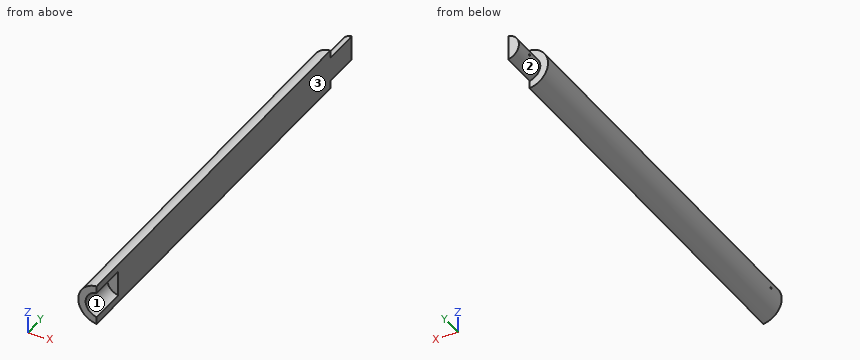
```python
from build123d import *

# Parameters (mm, degrees)
BOSS_EXTRUDE1_DEPTH     = 216.66667
BOSS_EXTRUDE2_START     = 216.66667
BOSS_EXTRUDE2_DEPTH     = 19.8
CUT_EXTRUDE2_START      = -1.4
SKETCH4_R               = 0.5
CUT_EXTRUDE2_DEPTH      = 9
SKETCH6_R               = 7
CUT_EXTRUDE3_DEPTH      = 20
CUT_EXTRUDE4_DEPTH      = 237.977817671
CUT_EXTRUDE4_DEPTH_BACK = 20
SKETCH7_R               = 0.5
CUT_EXTRUDE5_DEPTH      = 237.97781768
CUT_EXTRUDE5_DEPTH_BACK = 237.97781768
SKETCH10_R              = 0.5
CUT_EXTRUDE6_DEPTH      = 237.97781768
CUT_EXTRUDE6_DEPTH_BACK = 237.97781768
SKETCH11_W              = 3.5
SKETCH11_H              = 216.66667
CUT_EXTRUDE7_DEPTH      = 237.975709212
CUT_EXTRUDE7_DEPTH_BACK = 237.975709212
SKETCH12_W              = 3.499316008
SKETCH12_H              = 20


with BuildPart() as part:
    # Sketch1 → Boss-Extrude1 (new body)
    with BuildSketch(Plane(origin=(0, 0, 0), x_dir=(1, 0, 0), z_dir=(0, 1, 0))):
        with BuildLine():
            Line((0, 11), (0, -11))
            ThreePointArc((0, -11), (-11, 0), (0, 11))
        make_face()
    extrude(amount=BOSS_EXTRUDE1_DEPTH)

    # Sketch2 → Boss-Extrude2 (add)
    with BuildSketch(Plane(origin=(0, 0, 0), x_dir=(1, 0, 0), z_dir=(0, 1, 0)).offset(BOSS_EXTRUDE2_START)):
        with BuildLine():
            Line((0, 6.8), (0, -6.8))
            ThreePointArc((0, -6.8), (-6.8, 0), (0, 6.8))
        make_face()
    extrude(amount=BOSS_EXTRUDE2_DEPTH)

    # Sketch4 → Cut-Extrude2 (cut)
    with BuildSketch(Plane(origin=(0, 0, 0), x_dir=(0, 0, -1), z_dir=(1, 0, 0)).offset(CUT_EXTRUDE2_START)):
        with Locations((0, 226.66667)):
            Circle(SKETCH4_R)
    extrude(amount=-CUT_EXTRUDE2_DEPTH, mode=Mode.SUBTRACT)

    # Sketch6 → Cut-Extrude3 (cut)
    with BuildSketch(Plane(origin=(0, 0, 0), x_dir=(1, 0, 0), z_dir=(0, 1, 0))):
        Circle(SKETCH6_R)
    extrude(amount=CUT_EXTRUDE3_DEPTH, mode=Mode.SUBTRACT)

    # Sketch7 → Cut-Extrude4 (cut, two sides: drawn at the far end of the back side and taken through both)
    with BuildSketch(Plane(origin=(0, 0, 0), x_dir=(0, 0, -1), z_dir=(1, 0, 0)).offset(-CUT_EXTRUDE4_DEPTH_BACK)):
        with Locations(Location((0, 10, 0), (0, 0, 180))):
            Circle(SKETCH7_R)
    extrude(amount=CUT_EXTRUDE4_DEPTH + CUT_EXTRUDE4_DEPTH_BACK, mode=Mode.SUBTRACT)

    # Sketch10 → Cut-Extrude5 (cut, two sides: drawn at the far end of the back side and taken through both)
    with BuildSketch(Plane.XY.offset(-CUT_EXTRUDE5_DEPTH_BACK)):
        with Locations((0, 5)):
            Circle(SKETCH10_R)
    extrude(amount=CUT_EXTRUDE5_DEPTH + CUT_EXTRUDE5_DEPTH_BACK, mode=Mode.SUBTRACT)

    # Sketch11 → Cut-Extrude6 (cut, two sides: drawn at the far end of the back side and taken through both)
    with BuildSketch(Plane.XY.offset(-CUT_EXTRUDE6_DEPTH_BACK)):
        with Locations((0.750341996, 108.333335)):
            Rectangle(SKETCH11_W, SKETCH11_H)
    extrude(amount=CUT_EXTRUDE6_DEPTH + CUT_EXTRUDE6_DEPTH_BACK, mode=Mode.SUBTRACT)

    # Sketch12 → Cut-Extrude7 (cut, two sides: drawn at the far end of the back side and taken through both)
    with BuildSketch(Plane.XY.offset(-CUT_EXTRUDE7_DEPTH_BACK)):
        with Locations((0.75, 226.66667)):
            Rectangle(SKETCH12_W, SKETCH12_H)
    extrude(amount=CUT_EXTRUDE7_DEPTH + CUT_EXTRUDE7_DEPTH_BACK, mode=Mode.SUBTRACT)


solid = part.part
```
Here's how the part is built. I have some questions about the finished solid (model axes, mm). Face numbers are marked on the shaded views. Coordinates: 2 decimals unless noted, no trailing zeros. Order: outer loops, then holes, each group sorted by start corner. A loop starts at its lowest first (then second) coordinate and runs counter-clockwise, first axis right, second up. Notation, with made-up numbers: (67.25, -1) - (89.25, -1) arc R11 ccw to (89.25, 13) - close; hole circle Ø3 at (49, -13.75). An arc over 180 degrees is marked (long way). One line per question, with ' | ' between items.
(1) If I drill on L1, parallel to Y at x = -5.35, z = 0; L2, parallel to Y at x = -8, z = 0; L3, parallel to Z at x = -4, y = 19, over which ranges is the centre line in solid material (lowest first)?
Report:
L1: y = 20 to 226.17, 227.17 to 236.47 | L2: y = 0 to 9.5, 10.5 to 216.67 | L3: z = -10.25 to -5.74, 5.74 to 10.25
(2) Suppose I cut it at D-D on z = -4.5. List the corners of the cut face in (x, y) for me, and give its area (3 significant figures).
Report:
outline: (-10.04, 0) - (-5.36, 0) - (-5.36, 20) - (-1, 20) - (-1, 236.47) - (-5.1, 236.47) - (-5.1, 216.67) - (-10.04, 216.67) - close | area: 1,950 mm2
(3) Suppose I cut it at A-A on x = -3.5. List the corners of the cut face in (y, z) for me.
Report:
outline: (0, -10.43) - (216.67, -10.43) - (216.67, -5.83) - (236.47, -5.83) - (236.47, 5.83) - (216.67, 5.83) - (216.67, 10.43) - (0, 10.43) - (0, 6.06) - (20, 6.06) - (20, -6.06) - (0, -6.06) - close; hole circle Ø1 at (226.67, 0)
(4) If we mould it in two halves opening along Z, with no side actions, what happens to the marked faces 1, 2 and 3? For each: pulls with the +Z half, pulls with the -Z half, needs draft (parallel to the pull), parting line crosses it, or undercut.
Report:
face 1: undercut | face 2: parting line crosses it | face 3: needs draft
(5) Will these pins go through, and if not, where does the flat tip stop? pin 1 (2 mm diameter, centred on y = 121, z = -2.5, fed in from -X); pin 2 (3 mm diameter, centred on x = -8, z = 2.5, fed in from +Y); pin 3 (5 mm diameter, centred on x = -8.5, y = 72.5, fed in from +Z).
Report:
pin 1: stops at x = -10.9 | pin 2: stops at y = 216.67 | pin 3: stops at z = 9.22
(6) Suppose I cut it at C-C on z = 4.25. List the corners of the cut face in (x, y) for me, and give its area (3 significant figures).
Report:
outline: (-10.15, 0) - (-5.56, 0) - (-5.56, 20) - (-1, 20) - (-1, 236.47) - (-5.31, 236.47) - (-5.31, 216.67) - (-10.15, 216.67) - close | area: 1,980 mm2
